```python
from build123d import *

# Parameters (mm, degrees)
EXTRUDE_1_DEPTH      = 1
EXTRUDE_1_DEPTH_BACK = 1
SKETCH_1_W           = 10
SKETCH_1_H           = 1.5
SKETCH_2_R           = 0.4
EXTRUDE_2_DEPTH      = 0.2


with BuildPart() as part:
    # 草图1 → 凸台-拉伸1 (new, two sides: drawn at the far end of the back side and taken through both)
    with BuildSketch(Plane.XY.offset(-EXTRUDE_1_DEPTH_BACK)):
        with Locations((5, 0.75)):
            Rectangle(SKETCH_1_W, SKETCH_1_H)
    extrude(amount=EXTRUDE_1_DEPTH + EXTRUDE_1_DEPTH_BACK)

    # 草图2 → 凸台-拉伸2 (add)
    with BuildSketch(Plane.XY.offset(1)):
        with Locations((9, -0.2)):
            Circle(SKETCH_2_R)
        with Locations((1, -0.2)):
            Circle(SKETCH_2_R)
    extrude_2 = extrude(amount=-EXTRUDE_2_DEPTH)

    # 镜向1: 凸台-拉伸2 across plane
    add(extrude_2.mirror(Plane.XY))


solid = part.part
```
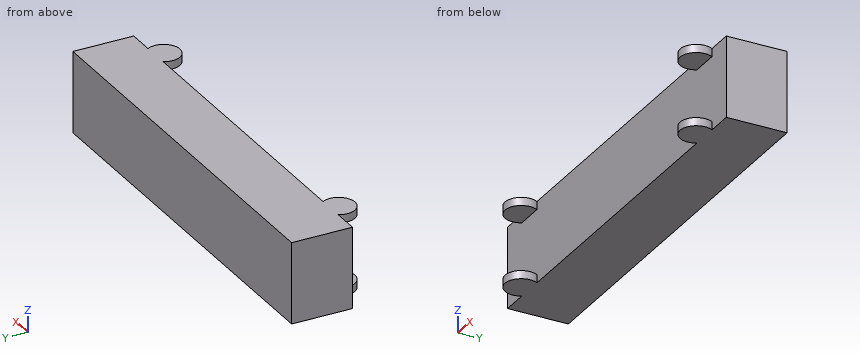
Geometry check sheet. Reference: the model listing, model coordinates, mm. Give positions to 0.01 mm unless a question says otherwise; leave off trailing zeros. Write each loop counter-clockwise with the first axis right and the second up, starting at its lowest first coordinate (ties: lowest second). Pieces come first, ordered by that corner, then holes. Notation, with made-up numbers: (-28.75, 12) -> (-7.75, 12) arc R27 ccw to (-7.75, 38) -> close; hole circle Ø6 at (58.25, 34.5). An arc over 180 degrees is marked (long way). Use one line per item in the form item = value.
Item 1: Scan lines: line 1 (Y direction, x = 1, z = 0.4); line 2 (X direction, y = -0.15, z = 0.95). Record each from-to range of solid material in increasing order.
Results list:
line_1 = 0 to 1.5
line_2 = 0.6 to 1.4, 8.6 to 9.4
Item 2: Sectioned sample at D-D on x = 8.75. Enter the section's corners in (y, z).
Results list:
outline = (-0.51, -1) -> (1.5, -1) -> (1.5, 1) -> (-0.51, 1) -> (-0.51, 0.8) -> (0, 0.8) -> (0, -0.8) -> (-0.51, -0.8) -> close
Item 3: Sectioned sample at B-B on x = 1. Enter the section's corners in (y, z), plus the area to 3 significant figures.
Results list:
outline = (-0.6, -1) -> (1.5, -1) -> (1.5, 1) -> (-0.6, 1) -> (-0.6, 0.8) -> (0, 0.8) -> (0, -0.8) -> (-0.6, -0.8) -> close
area = 3.24 mm2
Item 4: Sectioned sample at A-A on y = -0.2. Enter the section's corners in (x, z), plus the area to 3 significant figures.
Results list:
outline = (0.6, -1) -> (1.4, -1) -> (1.4, -0.8) -> (0.6, -0.8) -> close; (0.6, 0.8) -> (1.4, 0.8) -> (1.4, 1) -> (0.6, 1) -> close; (8.6, -1) -> (9.4, -1) -> (9.4, -0.8) -> (8.6, -0.8) -> close; (8.6, 0.8) -> (9.4, 0.8) -> (9.4, 1) -> (8.6, 1) -> close
area = 0.640 mm2
Item 5: Depth check by flat-ended pin: pin 1 Ø1 at (x, z) = (6, 0) entering from -Y; pin 2 Ø1 at (y, z) = (0.5, 0) entering from -X. Enter the tip coordinate at first touch or a pass-through.
Results list:
pin_1 = 0
pin_2 = 0
Item 6: Sectioned sample at C-C on z = 0. Enter the section's corners in (x, y), plus the area to 3 significant figures.
Results list:
outline = (0, 0) -> (10, 0) -> (10, 1.5) -> (0, 1.5) -> close
area = 15.0 mm2
